from build123d import *

# Parameters (mm, degrees)
F0_W     = 6.3244109941
F0_H     = 2
F1_DEPTH = 1
F2_DEPTH = 1
F3_W     = 7.2049933622
F3_H     = 2
F4_DEPTH = 1
F5_SIZE2 = 0.99999
F5_SIZE  = 1.59999


# Not quite as in the source:
# - a fillet or chamfer is up to 0.001 mm smaller than in the source, because OpenCascade refuses the exact size


with BuildPart() as f1:
    # F0 (on Top) → F1 (new body)
    with BuildSketch(Plane.XY):
        Polygon((-13.5638297198, 2), (-23.5638297198, 2), (-23.5638297198, 0), (-21.6967508232, 0), (-15.3723398291, 0), (-13.5638297198, 0), align=None)
        with Locations((-18.5345453261, -1)):
            Rectangle(F0_W, F0_H)
    extrude(amount=F1_DEPTH)

    # F0 (on Top) → F2 (join)
    with BuildSketch(Plane.XY):
        Polygon((-13.5638297198, 2), (-23.5638297198, 2), (-23.5638297198, 0), (-21.6967508232, 0), (-15.3723398291, 0), (-13.5638297198, 0), align=None)
    extrude(amount=-F2_DEPTH)

    # F3 (on face) → F4 (join)
    with BuildSketch(Plane(origin=(0, 0, -1), x_dir=(1, 0, 0), z_dir=(0, 0, -1))):
        with Locations((-18.5119810809, 2.8)):
            Rectangle(F3_W, F3_H)
    extrude(amount=-F4_DEPTH)

    # F5 (size 1.6 and 1 in the source; OpenCascade refuses exactly that, so slightly less here)
    f5_edges = [f1.edges().sort_by_distance(p)[0] for p in [
        (-18.511981, -3.8, 0),
    ]]
    f5_side = f1.faces().sort_by_distance((-18.50981, -2.886602, 0))[0]
    chamfer(f5_edges, length=F5_SIZE, length2=F5_SIZE2, reference=f5_side)


solid = f1.part
Verification items for the finished model (mm, model axes). A direction names the side the tool comes from. Give positions to 0.01 mm unless a question says otherwise; leave off trailing zeros. Loops run counter-clockwise (first coordinate to the right, second up) from the corner with the lowest first, then second, coordinate; pieces in that order, holes last.
1) Set-up check for faces 1 (the flat face through (-14.909, -2.6, -0.6)), 2 (the flat face through (-18.6, 0, -0.2)), 3 (the flat face through (-19, -1, 0)), 4 (the flat face through (-18, 2, 0)), 5 (the flat face through (-22.114, -2.6, -0.6)): record each of +Z, -Z, +X, -X, +Y, -Y from which the full face is reachable in a straight line by a thin tool's end or side.
2) Sectioned sample at A-A, the plane z = 0.85. Enter the section's corners in (x, y).
3) Depth check by flat-ended pin: pin 1 Ø1.1 at (y, z) = (-1.5, 0.5) entering from +X; pin 2 Ø0.5 at (y, z) = (-3, -0.5) entering from -X; pin 3 Ø0.5 at (y, z) = (-1, 0.5) entering from -X. Enter the tip coordinate at first touch or a pass-through.
4) Sectioned sample at B-B, the plane y = -1.9. Enter the section's corners in (x, z).
5) Draft check along Y on faces 6 (the flat face through (-13.564, 1, 0)), 7 (the flat face through (-18.6, -2, 0.5)), 8 (the flat face through (-18.6, -1.8, -0.5)). Enter one of: pulls with the +Y half, pulls with the -Y half, needs draft (parallel to the pull), parting line crosses it, or undercut.
6) Thickness scan on line 1 along X through (y, z) = (-1.7, 0.3); line 2 along Z through (x, y) = (-15.75, -0.1); line 3 along Y through (x, z) = (-18, 0.35). Record the ranges inside material, lowest first.
7) Sectioned sample at D-D, the plane z = -0.5. Enter the section's corners in (x, y).
Answers:
1. face 1: +Z, -Z, +X, -Y
1. face 2: -Z
1. face 3: -Z, +X, -X
1. face 4: +Z, -Z, +X, -X, +Y
1. face 5: +Z, -Z, -X, -Y
2. outline: (-23.56, 0) - (-21.7, 0) - (-21.7, -2) - (-15.37, -2) - (-15.37, 0) - (-13.56, 0) - (-13.56, 2) - (-23.56, 2) - close
3. pin 1: stops at x = -15.37
3. pin 2: stops at x = -22.11
3. pin 3: stops at x = -21.7
4. outline: (-22.11, -1) - (-14.91, -1) - (-14.91, 0) - (-15.37, 0) - (-15.37, 1) - (-21.7, 1) - (-21.7, 0) - (-22.11, 0) - close
5. face 6: needs draft
5. face 7: pulls with the -Y half
5. face 8: undercut
6. line 1: x = -21.7 to -15.37
6. line 2: z = 0 to 1
6. line 3: y = -2 to 2
7. outline: (-23.56, 0) - (-13.56, 0) - (-13.56, 2) - (-23.56, 2) - close; (-22.11, -3) - (-14.91, -3) - (-14.91, -1.8) - (-22.11, -1.8) - close
